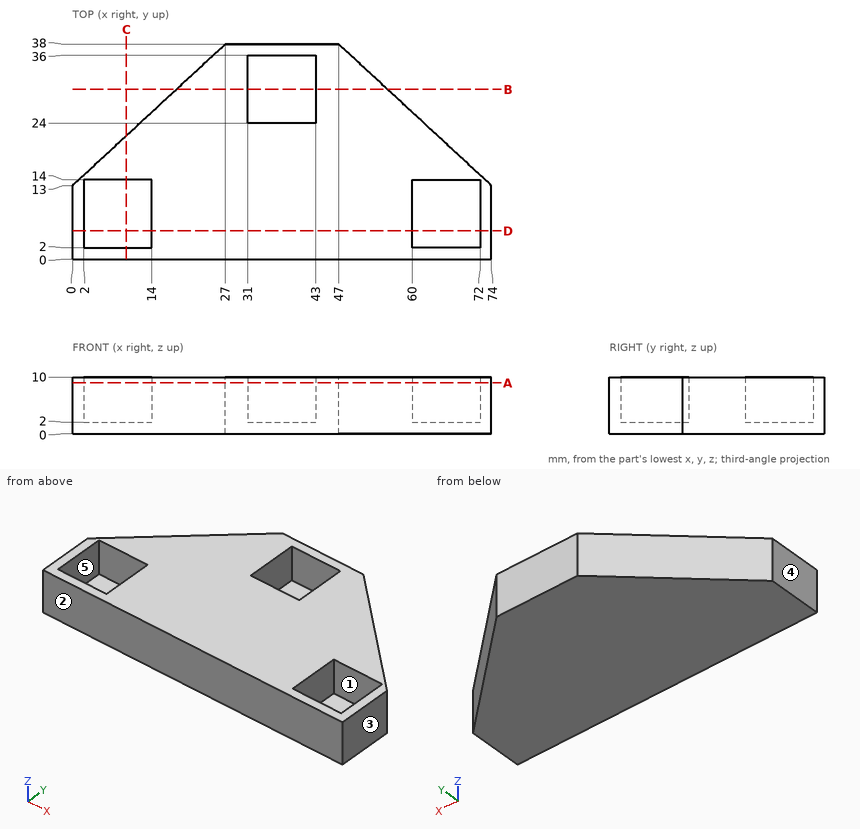
Drawing for the job (mm, zero at the part's lowest x, y, z). A direction names the side the tool comes from. Give positions to 0.01 mm unless a question says otherwise; leave off trailing zeros. Order: outer loops, then holes, each group sorted by start corner. A loop starts at its lowest first (then second) coordinate and runs counter-clockwise, first axis right, second up. Notation, with made-up numbers: (80.25, 31) - (86.25, 31) arc R23 ccw to (86.25, 58) - close; hole circle Ø11 at (43, -29). An arc over 180 degrees is marked (long way). Use one line per item in the form item = value.
Item 1: Pin check, flat tips, straight feed: pin 1 Ø6 at (x, y) = (10, 6.5) entering from +Z; pin 2 Ø5 at (y, z) = (34, 7) entering from -X; pin 3 Ø2.5 at (y, z) = (28.5, 5.5) entering from +X. Stop position of each tip, or through.
Solution:
pin_1 = 2
pin_2 = 19.98
pin_3 = 58.61
Item 2: Probe probe 1 along X at (y, z) = (11, 6); probe 2 along Y at (x, z) = (34, 5); probe 3 along Y at (x, z) = (10.5, 2.25). List the from-to ranges inside material, lowest first. Write a range as from..to.
Solution:
probe_1 = 0..2, 14..60, 72..74
probe_2 = 0..24, 36..38
probe_3 = 0..2, 14..22.72
Item 3: Slice it at C-C on x = 9.5. Give the cut face in (y, z), and give its area (3 significant figures).
Solution:
outline = (0, 0) - (21.8, 0) - (21.8, 10) - (14, 10) - (14, 2) - (2, 2) - (2, 10) - (0, 10) - close
area = 122 mm2
Item 4: Slice it at A-A on z = 9. Give the cut face in (x, y), and give its area (4 significant figures).
Solution:
outline = (0, 0) - (74, 0) - (74, 13) - (47, 38) - (27, 38) - (0, 13) - close; hole (2, 2) - (14, 2) - (14, 14) - (2, 14) - close; hole (31, 24) - (43, 24) - (43, 36) - (31, 36) - close; hole (60, 2) - (72, 2) - (72, 14) - (60, 14) - close
area = 1,705 mm2
Item 5: Which spindle directions (+Z, -Z, +X, -X, +Y, -Y) get a long thin tool onto all of the face, cutting with end or side? Do the marked faces 4 and 5. Say none if no direction does.
Solution:
face_4 = +Z, -Z, -X, +Y, -Y
face_5 = +Z
Item 6: Two-plate mould, pull along X, no slides. Class the marked faces 1, 2 and 3: released by +X, released by -X, zero draft, split by the parting line, or undercut.
Solution:
face_1 = undercut
face_2 = zero draft
face_3 = released by +X
Item 7: Slice it at B-B on y = 30. Give the cut face in (x, z).
Solution:
outline = (18.36, 0) - (55.64, 0) - (55.64, 10) - (43, 10) - (43, 2) - (31, 2) - (31, 10) - (18.36, 10) - close
Item 8: Slice it at D-D on y = 5. Give the cut face in (x, z), and give its area (3 significant figures).
Solution:
outline = (0, 0) - (74, 0) - (74, 10) - (72, 10) - (72, 2) - (60, 2) - (60, 10) - (14, 10) - (14, 2) - (2, 2) - (2, 10) - (0, 10) - close
area = 548 mm2
